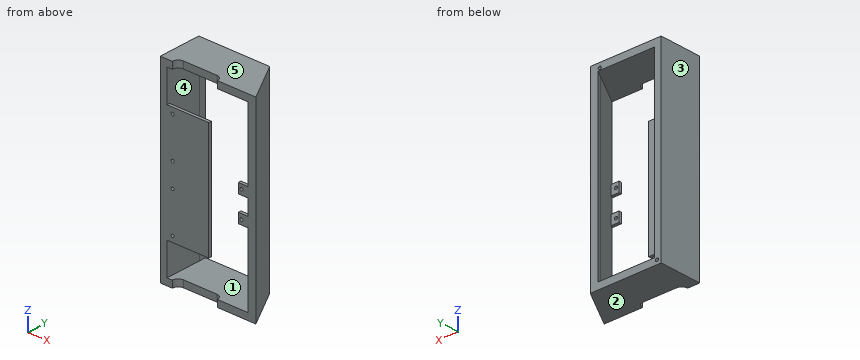
from build123d import *

# Parameters (mm, degrees)
BOSS_EXTRUDE1_DEPTH = 198
SHELL1_T            = -7
SKETCH2_W           = 184
SKETCH2_H           = 91.833810452
CUT_EXTRUDE1_DEPTH  = 10
SKETCH3_W           = 51.015734787
SKETCH3_H           = 184
CUT_EXTRUDE3_DEPTH  = 10
SKETCH4_W           = 43.227096231
SKETCH4_H           = 118.22
SKETCH4_W_2         = 10
SKETCH4_H_2         = 10
BOSS_EXTRUDE2_DEPTH = 3
SKETCH6_R           = 1.585
CUT_EXTRUDE5_DEPTH  = 10
SKETCH10_R          = 1.585
CUT_EXTRUDE8_DEPTH  = 5
SKETCH9_W           = 46.592666587
SKETCH9_H           = 6.179476357
CUT_EXTRUDE7_DEPTH  = 10
FILLET1_R           = 6
FILLET2_R           = 6
SKETCH11_R          = 1.585
CUT_EXTRUDE9_DEPTH  = 5
SKETCH12_R          = 1.585
CUT_EXTRUDE10_DEPTH = 5


with BuildPart() as part:
    # Sketch1 → Boss-Extrude1 (new body)
    with BuildSketch(Plane.XY):
        Polygon((0, 0), (99.07, 0), (73.665, 44.002750766), (0, 44.1), align=None)
    extrude(amount=BOSS_EXTRUDE1_DEPTH)

    # Shell1
    shell1_openings = [part.faces().sort_by_distance(p)[0] for p in [
        (49.535, 0, 99),
    ]]
    offset(amount=SHELL1_T, openings=shell1_openings, kind=Kind.INTERSECTION)

    # Sketch2 → Cut-Extrude1 (cut)
    with BuildSketch(Plane(origin=(68.240322174, 39.398568376, 0), x_dir=(0, 0, 1), z_dir=(-0.866025403784436, -0.5000000000000048, 0))):
        with Locations((99, 0.42335711)):
            Rectangle(SKETCH2_W, SKETCH2_H)
    extrude(amount=CUT_EXTRUDE1_DEPTH, mode=Mode.SUBTRACT)

    # Sketch3 → Cut-Extrude3 (cut)
    with BuildSketch(Plane(origin=(0.058218743, 44.099923142, 0), x_dir=(0.9999991285962467, -0.001320154061894519, 0), z_dir=(0.001320154061894519, 0.9999991285962467, 0))):
        with Locations((32.507861294, -99)):
            Rectangle(SKETCH3_W, SKETCH3_H)
    extrude(amount=-CUT_EXTRUDE3_DEPTH, mode=Mode.SUBTRACT)

    # Sketch4 → Boss-Extrude2 (add)
    with BuildSketch(Plane.XZ):
        with Locations((28.613548116, 99)):
            Rectangle(SKETCH4_W, SKETCH4_H)
        with Locations((85.987096231, 86)):
            Rectangle(SKETCH4_W_2, SKETCH4_H_2)
    boss_extrude2 = extrude(amount=-BOSS_EXTRUDE2_DEPTH)

    # Sketch6 → Cut-Extrude5 (cut)
    with BuildSketch(Plane(origin=(0, 3, 0), x_dir=(1, 0, 0), z_dir=(0, 1, 0))):
        with Locations(Location((12.830469551, -45.887182752, 0), (0, 0, 270))):
            Circle(SKETCH6_R)
        with Locations(Location((12.830469551, -86.887182752, 0), (0, 0, 270))):
            Circle(SKETCH6_R)
        with Locations(Location((12.830469551, -111.112817248, 0), (0, 0, 270))):
            Circle(SKETCH6_R)
        with Locations(Location((12.830469551, -152.112817248, 0), (0, 0, 270))):
            Circle(SKETCH6_R)
    extrude(amount=-CUT_EXTRUDE5_DEPTH, mode=Mode.SUBTRACT)

    # Sketch10 → Cut-Extrude8 (cut)
    with BuildSketch(Plane.XZ):
        with Locations(Location((84.092666587, 85.739056505, 0), (0, 0, 270))):
            Circle(SKETCH10_R)
    cut_extrude8 = extrude(amount=-CUT_EXTRUDE8_DEPTH, mode=Mode.SUBTRACT)

    # Sketch9 → Cut-Extrude7 (cut)
    with BuildSketch(Plane.XY.offset(198)):
        with Locations((35.796333293, 3.089738179)):
            Rectangle(SKETCH9_W, SKETCH9_H)
    cut_extrude7 = extrude(amount=-CUT_EXTRUDE7_DEPTH, mode=Mode.SUBTRACT)

    # Mirror1: Cut-Extrude7 across plane
    add(cut_extrude7.mirror(Plane(origin=(0, 0, 99), x_dir=(1, 0, 0), z_dir=(0, 0, -1))), mode=Mode.SUBTRACT)

    # Fillet1
    fillet1_edges = [part.edges().sort_by_distance(p)[0] for p in [
        (12.5, 6.179476357, 3.5),
        (59.092666587, 6.179476357, 3.5),
    ]]
    fillet(fillet1_edges, radius=FILLET1_R)

    # Fillet2
    fillet2_edges = [part.edges().sort_by_distance(p)[0] for p in [
        (12.5, 6.179476357, 194.5),
        (59.092666587, 6.179476357, 194.5),
    ]]
    fillet(fillet2_edges, radius=FILLET2_R)

    # Mirror2: Boss-Extrude2, Cut-Extrude8 across plane
    add(boss_extrude2.mirror(Plane(origin=(0, 0, 99), x_dir=(1, 0, 0), z_dir=(0, 0, -1))))
    add(cut_extrude8.mirror(Plane(origin=(0, 0, 99), x_dir=(1, 0, 0), z_dir=(0, 0, -1))), mode=Mode.SUBTRACT)

    # Sketch11 → Cut-Extrude9 (cut)
    with BuildSketch(Plane.XZ):
        with Locations(Location((12.830469551, 152.112817248, 0), (0, 0, 270))):
            Circle(SKETCH11_R)
        with Locations(Location((12.830469551, 111.112817248, 0), (0, 0, 270))):
            Circle(SKETCH11_R)
        with Locations(Location((12.830469551, 86.887182752, 0), (0, 0, 270))):
            Circle(SKETCH11_R)
        with Locations(Location((12.830469551, 45.887182752, 0), (0, 0, 270))):
            Circle(SKETCH11_R)
    extrude(amount=-CUT_EXTRUDE9_DEPTH, mode=Mode.SUBTRACT)

    # Sketch12 → Cut-Extrude10 (cut)
    with BuildSketch(Plane(origin=(0.058218743, 44.099923142, 0), x_dir=(0.9999991285962467, -0.001320154061894519, 0), z_dir=(0.001320154061894519, 0.9999991285962467, 0))):
        with Locations(Location((63.768297777, -193.245706001, 0), (0, 0, 180))):
            Circle(SKETCH12_R)
        with Locations(Location((4.416986766, -4.402159503, 0), (0, 0, 180))):
            Circle(SKETCH12_R)
    extrude(amount=-CUT_EXTRUDE10_DEPTH, mode=Mode.SUBTRACT)


solid = part.part
Model file for the job. Use its own axes, mm. Face numbers are marked on the shaded views. A direction names the side the tool comes from. Round coordinates to 2 decimals unless told otherwise and drop trailing zeros. Loops run counter-clockwise (first coordinate to the right, second up) from the corner with the lowest first, then second, coordinate; pieces in that order, holes last.
1. Band-saw the part on C-C, the plane y = 34. List the corners of the cut face in (x, z), and give its area (3 significant figures).
Check values:
outline: (0, 0) - (79.44, 0) - (79.44, 198) - (0, 198) - close; hole (7, 7) - (71.36, 7) - (71.36, 191) - (7, 191) - close
area: 3,890 mm2
2. Mould opens along X. For the marked faces 3, 4 and 5 say: +X half, -X half, draft (parallel to the pull), parting line (faces both ways), or undercut.
Check values:
face 3: -X half
face 4: undercut
face 5: draft
3. Wall check: probe 1 along Z at (x, y) = (48.5, 42); probe 2 along X at (y, z) = (21.5, 95); probe 3 along X at (y, z) = (28.5, 27). Give the ranges that are in metal, low to high.
Check values:
probe 1: z = 0 to 7, 191 to 198
probe 2: x = 0 to 7, 78.57 to 86.66
probe 3: x = 0 to 7, 74.53 to 82.62
4. Band-saw the part on B-B, the plane x = 46. List the corners of the cut face in (y, z).
Check values:
outline: (0, 39.89) - (3, 39.89) - (3, 158.11) - (0, 158.11) - close; (6.18, 0) - (44.04, 0) - (44.04, 7) - (6.18, 7) - close; (6.18, 191) - (44.04, 191) - (44.04, 198) - (6.18, 198) - close
5. Band-saw the part on D-D, the plane z = 143. List the corners of the cut face in (x, y) (3 decimals).
Check values:
outline: (0, 0) - (50.227, 0) - (50.227, 3) - (7, 3) - (7, 37.091) - (7.049, 37.091) - (7.058, 44.091) - (0, 44.1) - close; (65.576, 44.013) - (90.987, 0) - (99.07, 0) - (73.665, 44.003) - close
6. Tool access for the marked faces 1 and 2: list every direction of +Z, -Z, +X, -X, +Y, -Y with a clear straight run to the whole face (end or side of a thin tool).
Check values:
face 1: -Y
face 2: -Z, +X, -X, +Y, -Y
7. Drop flat-ended pins along their axis: P1, Ø13, axis at x = 26.5, z = 100.5, coming from the +Y side; P2, Ø3.5, axis at x = 84.09, z = 112.26, coming from the +Y side; P3, Ø4, axis at x = 73, z = 129, coming from the +Y side; P4, Ø2.5, axis at x = 12.83, z = 86.89, coming from the +Y side. Give the stop position or say it passes through.
Check values:
P1: stops at y = 3
P2: stops at y = 28.98
P3: stops at y = 44.01
P4: passes through
8. Band-saw the part on A-A, the plane z = 20. List the corners of the cut face in (x, y) (3 decimals).
Check values:
outline: (0, 0) - (7, 0) - (7, 37.091) - (7.049, 37.091) - (7.058, 44.091) - (0, 44.1) - close; (65.576, 44.013) - (90.987, 0) - (99.07, 0) - (73.665, 44.003) - close
